```python
from build123d import *


with BuildPart() as part:
    # Sketch2 → Revolve1 (revolve)
    with BuildSketch(Plane(origin=(0, 0, 0), x_dir=(0, 0, -1), z_dir=(1, 0, 0)), mode=Mode.PRIVATE) as revolve1_sk:
        with BuildLine():
            Line((3, 4), (-3, 4))
            ThreePointArc((-3, 4), (-3.353553391, 4.146446609), (-3.5, 4.5))
            Line((-3.5, 4.5), (-3.5, 6.495))
            Line((-3.5, 6.495), (-3.37, 6.625))
            Line((-3.37, 6.625), (-1.515544457, 6.625))
            ThreePointArc((-1.515544457, 6.625), (0, 5.75), (1.515544457, 6.625))
            Line((1.515544457, 6.625), (3.37, 6.625))
            Line((3.37, 6.625), (3.5, 6.495))
            Line((3.5, 6.495), (3.5, 4.5))
            ThreePointArc((3.5, 4.5), (3.353553391, 4.146446609), (3, 4))
        make_face()
    revolve(revolve1_sk.sketch.rotate(Axis((0, 0, 3.5), (0, 0, -1)), 90), axis=Axis((0, 0, 3.5), (0, 0, -1)))


solid = part.part
```
Could you check a few things on this model? Use its own coordinates, in mm. Coordinates: 2 decimals unless noted, no trailing zeros. Loops run counter-clockwise (first coordinate to the right, second up) from the corner with the lowest first, then second, coordinate; pieces in that order, holes last.
1) Imagine slicing it at A-A (x = 0). List the corners of the cut face in (y, z) for me (3 decimals), and give its area (3 significant figures).
Reported:
outline: (-6.625, -3.37) - (-6.495, -3.5) - (-4.5, -3.5) arc R0.5 ccw to (-4, -3) - (-4, 3) arc R0.5 ccw to (-4.5, 3.5) - (-6.495, 3.5) - (-6.625, 3.37) - (-6.625, 1.516) arc R1.75 cw to (-6.625, -1.516) - close; (4, -3) arc R0.5 ccw to (4.5, -3.5) - (6.495, -3.5) - (6.625, -3.37) - (6.625, -1.516) arc R1.75 cw to (6.625, 1.516) - (6.625, 3.37) - (6.495, 3.5) - (4.5, 3.5) arc R0.5 ccw to (4, 3) - close
area: 32.7 mm2
2) Thinking about a two-plate mould opening in X: for faces 1 (the face through (-0.86, -6.57, -2.46)), 2 (the face through (-0.867, 3.905, 0.042)), 3 (the face through (-1.53, -4.42, -3.5)), which applies, released by +X, released by -X, zero draft, split by the parting line, or undercut?
Reported:
face 1: split by the parting line
face 2: undercut
face 3: zero draft
3) Imagine slicing it at D-D (z = 0). List the corners of the cut face in (x, y) for me, and give its area (3 significant figures).
Reported:
outline: circle Ø11.5 at (0, 0); hole circle Ø8 at (0, 0)
area: 53.6 mm2
4) Will these pins go through, and if not, where does the flat tip stop? pin 1 Ø4 at (x, z) = (4, -2) entering from -Y; pin 2 Ø1 at (x, z) = (4, -0.5) entering from +Y; pin 3 Ø4 at (y, z) = (2.5, -2.5) entering from -X.
Reported:
pin 1: stops at y = -6.32
pin 2: stops at y = 4.73
pin 3: stops at x = -6.61
5) Imagine slicing it at C-C (z = 2.75). List the corners of the cut face in (x, y) for me (3 decimals), and give its area (3 significant figures).
Reported:
outline: circle Ø13.25 at (0, 0); hole circle Ø8 at (0, 0)
area: 87.6 mm2
6) Please list where these lines run through material, in increasing order: line 1 along Y through (x, z) = (0, 1.75) (3 decimals); line 2 along Y through (x, z) = (2.25, 1); line 3 along Z through (x, y) = (0.5, -6).
Reported:
line 1: y = -6.625 to -4, 4 to 6.625
line 2: y = -5.63 to -3.31, 3.31 to 5.63
line 3: z = -3.5 to -0.94, 0.94 to 3.5
